from build123d import *

# Parameters (mm, degrees)
SKETCH1_W                                            = 12.5
SKETCH1_H                                            = 2.9
CBORE_FOR_M2_5_HEX_SOCKET_HEAD_CAP_SCREW_D           = 2.9
CBORE_FOR_M2_5_HEX_SOCKET_HEAD_CAP_SCREW_CBORE_D     = 5.5
CBORE_FOR_M2_5_HEX_SOCKET_HEAD_CAP_SCREW_CBORE_DEPTH = 2.1
CIRPATTERN1_COUNT                                    = 6
CUT_EXTRUDE4_DEPTH                                   = 10
SKETCH5_R                                            = 39.98
SKETCH5_R_2                                          = 34
BOSS_EXTRUDE1_DEPTH                                  = 1


with BuildPart() as part:
    # Sketch1 → Revolve1 (revolve)
    with BuildSketch(Plane.XY):
        with Locations((-33.75, 1.45)):
            Rectangle(SKETCH1_W, SKETCH1_H)
    revolve(axis=Axis((0, -3.243860323, 0), (0, 1, 0)))

    # CBORE for M2.5 Hex Socket Head Cap Screw2 (through all)
    with Locations(Plane(origin=(0, 3.4, 0), x_dir=(-1, 0, 0), z_dir=(0, 1, 0))):
        with Locations((0, -30.75)):
            cbore_for_m2_5_hex_socket_head_cap_screw = CounterBoreHole(CBORE_FOR_M2_5_HEX_SOCKET_HEAD_CAP_SCREW_D / 2, CBORE_FOR_M2_5_HEX_SOCKET_HEAD_CAP_SCREW_CBORE_D / 2, CBORE_FOR_M2_5_HEX_SOCKET_HEAD_CAP_SCREW_CBORE_DEPTH)

    # CirPattern1: CBORE for M2.5 Hex Socket Head Cap Screw2 ×6 about axis
    cirpattern1_axis = Axis((0, 0, 0), (0, 1, 0))
    for i in range(1, CIRPATTERN1_COUNT):
        add(cbore_for_m2_5_hex_socket_head_cap_screw.rotate(cirpattern1_axis, i * 360 / CIRPATTERN1_COUNT), mode=Mode.SUBTRACT)

    # Sketch10 → Cut-Extrude4 (cut)
    with BuildSketch(Plane(origin=(0, 2.9, 0), x_dir=(1, 0, 0), z_dir=(0, 1, 0))):
        with BuildLine():
            Line((-32, 1.5), (-30, 1.5))
            ThreePointArc((-30, 1.5), (-28.5, 0), (-30, -1.5))
            Line((-30, -1.5), (-32, -1.5))
            ThreePointArc((-32, -1.5), (-33.5, 0), (-32, 1.5))
        make_face()
    extrude(amount=-CUT_EXTRUDE4_DEPTH, mode=Mode.SUBTRACT)

    # Sketch5 → Boss-Extrude1 (add)
    with BuildSketch(Plane(origin=(0, 2.9, 0), x_dir=(1, 0, 0), z_dir=(0, 1, 0))):
        Circle(SKETCH5_R)
        Circle(SKETCH5_R_2, mode=Mode.SUBTRACT)
    extrude(amount=BOSS_EXTRUDE1_DEPTH)


solid = part.part
Model file for the job. Use its own axes, mm. A direction names the side the tool comes from. Round coordinates to 2 decimals unless told otherwise and drop trailing zeros.
(1) Band-saw the part on A-A (z = 0). Give the number of separate pieces and of enclosed holes in the cut face, then the cut area to 3 significant figures.
(2) Pull direction X, two halves, no side cores. Call faces 3 (the face through (8.67, 1.47, -39.05)), 4 (the face through (-26.27, 2.11, 18.1)), 5 (the face through (-21, 3.9, -27)): released by +X, released by -X, zero draft, split by the parting line, or undercut.
(3) Drill centre lines: line 1 (Z direction, x = 0, y = 0.7); line 2 (Z direction, x = 0, y = 2.25); line 3 (Z direction, x = 0, y = 3.2). Where is each one in solid material? Low to high.
(4) 3-axis set-ups, long thin cutter, end or side, ignore diameter. For faces 1 (the face through (28.2, 1.3, 14.9)), 2 (the face through (-33.5, 1.5, 0)): which of +Z, -Z, +X, -X, +Y, -Y reach the whole face in a straight line?
(5) Pin check, flat tips, straight feed: pin 1 (1.6 mm diameter, centred on x = 27, z = 14, fed in from +Y); pin 2 (7 mm diameter, centred on x = -26.63, z = 15.37, fed in from -Y); pin 3 (2 mm diameter, centred on x = -30.5, y = 1, fed in from -Z); pin 4 (6 mm diameter, centred on x = -25.5, z = -14.5, fed in from +Y). Stop position of each tip, or through.
Verdict:
1. separate pieces: 3
1. enclosed holes: 0
1. area: 70.0 mm2
2. face 3: split by the parting line
2. face 4: undercut
2. face 5: zero draft
3. line 1: z = -40 to -32.2, -29.3 to -27.5, 27.5 to 29.3, 32.2 to 40
3. line 2: z = -40 to -33.5, -28 to -27.5, 27.5 to 28, 33.5 to 40
3. line 3: z = -39.98 to -34, 34 to 39.98
4. face 1: +Y
4. face 2: +Y, -Y
5. pin 1: stops at y = 1.3
5. pin 2: stops at y = 0
5. pin 3: stops at z = -27.01
5. pin 4: stops at y = 2.9
